Here's how the part is built. I have some questions about the finished solid (model axes, mm). A direction names the side the tool comes from. Round coordinates to 2 decimals unless told otherwise and drop trailing zeros. Write each loop counter-clockwise with the first axis right and the second up, starting at its lowest first coordinate (ties: lowest second). Pieces come first, ordered by that corner, then holes. Notation, with made-up numbers: (-13.75, 27) -> (33.25, 27) arc R26 cw to (33.25, 54) -> close; hole circle Ø5 at (-27, 19.25). An arc over 180 degrees is marked (long way). Answer in a Markdown table with one row per item.
from build123d import *

# Parameters (mm, degrees)
SKETCH1_W                = 60
SKETCH1_H                = 60
BOSS_EXTRUDE1_DEPTH      = 45
CUT_EXTRUDE1_DEPTH       = 30
FILLET1_R                = 3
SKETCH4_R                = 15
CUT_EXTRUDE2_DEPTH       = 46
M4_CLEARANCE_HOLE1_D     = 4.5
M4_CLEARANCE_HOLE1_DEPTH = 15
SKETCH6_R                = 3
CUT_EXTRUDE3_DEPTH       = 20
FILLET2_R                = 3
CHAMFER1_SIZE            = 0.5


with BuildPart() as part:
    # Sketch1 → Boss-Extrude1 (new body)
    with BuildSketch(Plane.XY):
        Rectangle(SKETCH1_W, SKETCH1_H)
    extrude(amount=BOSS_EXTRUDE1_DEPTH)

    # Sketch3 → Cut-Extrude1 (cut)
    with BuildSketch(Plane.XY.offset(45)):
        with BuildLine():
            ThreePointArc((-23.5712, 16.5712), (-18.621452532, 18.621452532), (-16.5712, 23.5712))
            Line((-16.5712, 23.5712), (-16.5712, 30))
            Line((-16.5712, 30), (-30, 30))
            Line((-30, 30), (-30, 16.5712))
            Line((-30, 16.5712), (-23.5712, 16.5712))
        make_face()
        with BuildLine():
            Line((30, 30), (16.5712, 30))
            Line((16.5712, 30), (16.5712, 23.5712))
            ThreePointArc((16.5712, 23.5712), (18.621452532, 18.621452532), (23.5712, 16.5712))
            Line((23.5712, 16.5712), (30, 16.5712))
            Line((30, 16.5712), (30, 30))
        make_face()
        with BuildLine():
            Line((30, -30), (30, -16.5712))
            Line((30, -16.5712), (23.5712, -16.5712))
            ThreePointArc((23.5712, -16.5712), (18.621452532, -18.621452532), (16.5712, -23.5712))
            Line((16.5712, -23.5712), (16.5712, -30))
            Line((16.5712, -30), (30, -30))
        make_face()
        with BuildLine():
            Line((-23.5712, -16.5712), (-30, -16.5712))
            Line((-30, -16.5712), (-30, -30))
            Line((-30, -30), (-16.5712, -30))
            Line((-16.5712, -30), (-16.5712, -23.5712))
            ThreePointArc((-16.5712, -23.5712), (-18.621452532, -18.621452532), (-23.5712, -16.5712))
        make_face()
    extrude(amount=-CUT_EXTRUDE1_DEPTH, mode=Mode.SUBTRACT)

    # Fillet1
    fillet1_edges = [part.edges().sort_by_distance(p)[0] for p in [
        (-30, 30, 7.5),
        (30, 30, 7.5),
        (30, -30, 7.5),
        (-30, -30, 7.5),
    ]]
    fillet(fillet1_edges, radius=FILLET1_R)

    # Sketch4 → Cut-Extrude2 (cut, through all)
    with BuildSketch(Plane.XY.offset(45)):
        Circle(SKETCH4_R)
    extrude(amount=-CUT_EXTRUDE2_DEPTH, mode=Mode.SUBTRACT)

    # M4 Clearance Hole1
    with Locations(Plane(origin=(-23.5712, 23.5712, 15), x_dir=(1, 0, 0), z_dir=(0, 0, 1))):
        with Locations((0, 0), (47.1424, 0), (47.1424, -47.1424), (0, -47.1424)):
            Hole(M4_CLEARANCE_HOLE1_D / 2, depth=M4_CLEARANCE_HOLE1_DEPTH)

    # Sketch6 → Cut-Extrude3 (cut)
    with BuildSketch(Plane.XY.offset(45)):
        with Locations((-15, 15)):
            Circle(SKETCH6_R)
        with Locations((-15, -15)):
            Circle(SKETCH6_R)
        with Locations((15, -15)):
            Circle(SKETCH6_R)
        with Locations((15, 15)):
            Circle(SKETCH6_R)
    extrude(amount=-CUT_EXTRUDE3_DEPTH, mode=Mode.SUBTRACT)

    # Fillet2
    fillet2_edges = [part.edges().sort_by_distance(p)[0] for p in [
        (-16.5712, 30, 30),
        (-30, 16.5712, 30),
        (30, 16.5712, 30),
        (16.5712, 30, 30),
        (16.5712, -30, 30),
        (30, -16.5712, 30),
        (-30, -16.5712, 30),
        (-16.5712, -30, 30),
    ]]
    fillet(fillet2_edges, radius=FILLET2_R)

    # Chamfer1
    chamfer1_edges = [part.edges().sort_by_distance(p)[0] for p in [
        (-15, 0, 45),
        (-18, 15, 45),
        (-18, -15, 45),
        (12, -15, 45),
        (12, 15, 45),
        (-30, 0, 45),
        (0, -30, 45),
        (30, 0, 45),
        (0, 30, 45),
        (-29.121320344, -15.692520344, 45),
        (-15.692520344, -29.121320344, 45),
        (15.692520344, -29.121320344, 45),
        (29.121320344, -15.692520344, 45),
        (29.121320344, 15.692520344, 45),
        (15.692520344, 29.121320344, 45),
        (-15.692520344, 29.121320344, 45),
        (-29.121320344, 15.692520344, 45),
        (-16.5712, 25.2856, 45),
        (-25.2856, 16.5712, 45),
        (-18.621452532, 18.621452532, 45),
        (18.621452532, 18.621452532, 45),
        (25.2856, 16.5712, 45),
        (16.5712, 25.2856, 45),
        (18.621452532, -18.621452532, 45),
        (16.5712, -25.2856, 45),
        (25.2856, -16.5712, 45),
        (-25.2856, -16.5712, 45),
        (-16.5712, -25.2856, 45),
        (-18.621452532, -18.621452532, 45),
    ]]
    chamfer(chamfer1_edges, length=CHAMFER1_SIZE)


solid = part.part
1) I want a section at A-A, the plane y = 0. List the corners of the cut face in (x, z) for me, and give its area (3 significant figures).
Response:
| item | result |
|---|---|
| outline | (-30, 0) -> (-15, 0) -> (-15, 44.5) -> (-15.5, 45) -> (-29.5, 45) -> (-30, 44.5) -> close; (15, 0) -> (30, 0) -> (30, 44.5) -> (29.5, 45) -> (15.5, 45) -> (15, 44.5) -> close |
| area | 1,350 mm^2 |
2) Which directions (+Z, -Z, +X, -X, +Y, -Y) give clear straight access to the entire face, cutting with the end or side of a thin tool? Please do faces 1 (the face through (15.669, -29.145, 29.544)), 2 (the face through (-29.145, 15.669, 29.544)), 3 (the face through (29.145, 15.669, 29.544)), 4 (the face through (-26, -25, 15)).
Response:
| item | result |
|---|---|
| face 1 | +Z, +X, -Y |
| face 2 | +Z, -X, +Y |
| face 3 | +Z, +X, +Y |
| face 4 | +Z, -X, -Y |
3) I need wall thicknesses on line 1 (Y direction, x = 0, z = 32); line 2 (Y direction, x = 27, z = 30); line 3 (X direction, y = 8, z = 15). Which ranges of each line are inside material? Lowest first, please. Write a range as [from, to].
Response:
| item | result |
|---|---|
| line 1 | y = [-30, -15], [15, 30] |
| line 2 | y = [-16.57, 16.57] |
| line 3 | x = [-30, -12.69], [12.69, 30] |
4) I want a section at B-B, the plane z = 22. List the corners of the cut face in (x, y) for me.
Response:
| item | result |
|---|---|
| outline | (-30, -13.57) arc R3 ccw to (-27, -16.57) -> (-23.57, -16.57) arc R7 cw to (-16.57, -23.57) -> (-16.57, -27) arc R3 ccw to (-13.57, -30) -> (13.57, -30) arc R3 ccw to (16.57, -27) -> (16.57, -23.57) arc R7 cw to (23.57, -16.57) -> (27, -16.57) arc R3 ccw to (30, -13.57) -> (30, 13.57) arc R3 ccw to (27, 16.57) -> (23.57, 16.57) arc R7 cw to (16.57, 23.57) -> (16.57, 27) arc R3 ccw to (13.57, 30) -> (-13.57, 30) arc R3 ccw to (-16.57, 27) -> (-16.57, 23.57) arc R7 cw to (-23.57, 16.57) -> (-27, 16.57) arc R3 ccw to (-30, 13.57) -> close; hole circle Ø30 at (0, 0) |
5) We'd pull the mould along X, two halves only. Please class faces 5 (the face through (-16.571, -25, 30)), 6 (the face through (12.6, 13.2, 34.9)), 7 (the face through (15, -15, 25)), 8 (the face through (28.843, 15.455, 44.865)): +X half, -X half, draft (parallel to the pull), parting line (faces both ways), or undercut.
Response:
| item | result |
|---|---|
| face 5 | -X half |
| face 6 | undercut |
| face 7 | undercut |
| face 8 | +X half |
6) I want a section at D-D, the plane z = 8. List the corners of the cut face in (x, y) for me.
Response:
| item | result |
|---|---|
| outline | (-30, -27) arc R3 ccw to (-27, -30) -> (27, -30) arc R3 ccw to (30, -27) -> (30, 27) arc R3 ccw to (27, 30) -> (-27, 30) arc R3 ccw to (-30, 27) -> close; hole circle Ø4.5 at (-23.57, -23.57); hole circle Ø4.5 at (-23.57, 23.57); hole circle Ø30 at (0, 0); hole circle Ø4.5 at (23.57, -23.57); hole circle Ø4.5 at (23.57, 23.57) |
7) For pin 1 (1.7 mm diameter, centred on x = -26, z = 26, fed in from -Y); pin 2 (5 mm diameter, centred on x = -15, y = -15, fed in from +Z); pin 3 (2.5 mm diameter, centred on y = 25, z = 35, fed in from -X); pin 4 (2.5 mm diameter, centred on x = 23.57, y = -23.57, fed in from +Z), each with a flat end and sliding along its axis, tell me the tip position at first contact or that it passes through.
Response:
| item | result |
|---|---|
| pin 1 | stops at y = -16.57 |
| pin 2 | stops at z = 25 |
| pin 3 | stops at x = -16.57 |
| pin 4 | passes through |
